For this review, take the finished solid that the model builds, in its own axes (mm). Round coordinates to 2 decimals unless told otherwise and drop trailing zeros. Order: outer loops, then holes, each group sorted by start corner. A loop starts at its lowest first (then second) coordinate and runs counter-clockwise, first axis right, second up. Notation, with made-up numbers: (-7.75, 53) - (29.25, 53) arc R14 cw to (29.25, 76) - close; hole circle Ø10 at (68, 24.5). An arc over 180 degrees is marked (long way). Write each question's results on one line, items separated by ' | '. Start each with the question number.
(1) Take a section at C-C, the plane x = 7.5. Give the boundary of the cut face in (y, z), plus the area to 3 significant figures.
(2) For L1, parallel to Z at x = -20.32, y = 0.15; L2, parallel to X at y = 0.4, z = 17.78; L3, parallel to X at y = -0.55, z = 15 (3 decimals), list the stretches that pass through material, from the lowest coordinate up. Write a range as from..to.
(3) Insertion check: pin 1 Ø4 at (x, z) = (-20.32, -17.78) entering from -Y; pin 2 Ø0.5 at (x, y) = (8, 0.5) entering from +Z; pin 3 Ø0.8 at (x, y) = (0, 0.5) entering from -Z; pin 4 Ø0.8 at (x, y) = (-7.5, 0) entering from -Z. Each pin has a flat end and moves straight along its axis. Give the tip position at first contact, or say it passes through.
(4) Take a section at B-B, the plane y = -0.4. Give the boundary of the cut face in (x, z) (3 decimals), plus the area to 3 significant figures.
(5) Take a section at A-A, the plane z = -14.5. Give the boundary of the cut face in (x, y) (3 decimals), plus the area to 3 significant figures.
```python
from build123d import *

# Parameters (mm, degrees)
SKETCH1_W             = 45.72
SKETCH1_H             = 40.64
BOSS_EXTRUDE1_DEPTH   = 0.762
FILLET1_R             = 2.54
F_4_CLEARANCE_HOLE1_D = 2.9464
SKETCH4_W             = 1.515
SKETCH4_H             = 4
CUT_EXTRUDE1_DEPTH    = 2.524


with BuildPart() as part:
    # Sketch1 → Boss-Extrude1 (new body, symmetric)
    with BuildSketch(Plane(origin=(0, 0, 0), x_dir=(1, 0, 0), z_dir=(0, 1, 0))):
        Rectangle(SKETCH1_W, SKETCH1_H)
    extrude(amount=BOSS_EXTRUDE1_DEPTH, both=True)

    # Fillet1
    fillet1_edges = [part.edges().sort_by_distance(p)[0] for p in [
        (22.86, 0, 20.32),
        (-22.86, 0, 20.32),
        (-22.86, 0, -20.32),
        (22.86, 0, -20.32),
    ]]
    fillet(fillet1_edges, radius=FILLET1_R)

    # #4 Clearance Hole1 (through all)
    with Locations(Plane(origin=(0, 0.762, 0), x_dir=(1, 0, 0), z_dir=(0, 1, 0))):
        with Locations((20.32, 17.78), (-20.32, -17.78), (-20.32, 17.78), (20.32, -17.78)):
            Hole(F_4_CLEARANCE_HOLE1_D / 2)

    # Sketch4 → Cut-Extrude1 (cut, through all)
    with BuildSketch(Plane(origin=(0, 0.762, 0), x_dir=(1, 0, 0), z_dir=(0, 1, 0))):
        Polygon((6.985, 16.32), (6.985, 20.32), (-6.985, 20.32), (-6.985, 16.32), (-6.985, 11.938), (6.985, 11.938), align=None)
        with Locations((7.7425, 18.32)):
            Rectangle(SKETCH4_W, SKETCH4_H)
        with Locations((-7.7425, 18.32)):
            Rectangle(SKETCH4_W, SKETCH4_H)
    cut_extrude1 = extrude(amount=-CUT_EXTRUDE1_DEPTH, mode=Mode.SUBTRACT)

    # Mirror1: Cut-Extrude1 across plane
    add(cut_extrude1.mirror(Plane.XY), mode=Mode.SUBTRACT)


solid = part.part
```
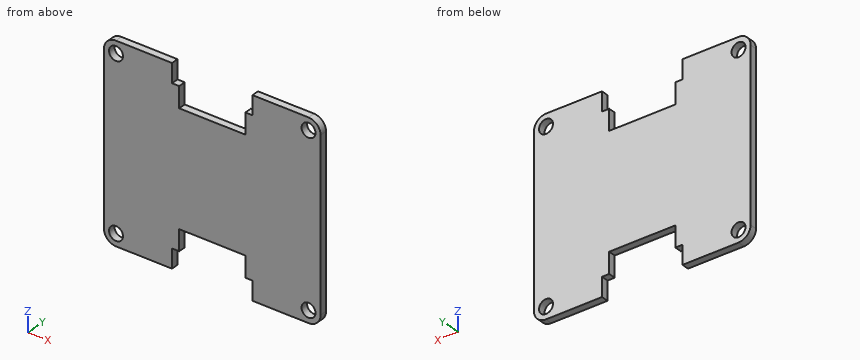
Results below:
1) outline: (-0.76, -16.32) - (0.76, -16.32) - (0.76, 16.32) - (-0.76, 16.32) - close | area: 49.7 mm^2
2) L1: z = -20.32..-19.25, -16.31..16.31, 19.25..20.32 | L2: x = -22.86..-21.79, -18.85..-8.5, 8.5..18.85, 21.79..22.86 | L3: x = -22.86..-6.985, 6.985..22.86
3) pin 1: stops at y = -0.76 | pin 2: stops at z = 16.32 | pin 3: stops at z = -11.94 | pin 4: stops at z = -16.32
4) outline: (-22.86, -17.78) arc R2.54 ccw to (-20.32, -20.32) - (-8.5, -20.32) - (-8.5, -16.32) - (-6.985, -16.32) - (-6.985, -11.938) - (6.985, -11.938) - (6.985, -16.32) - (8.5, -16.32) - (8.5, -20.32) - (20.32, -20.32) arc R2.54 ccw to (22.86, -17.78) - (22.86, 17.78) arc R2.54 ccw to (20.32, 20.32) - (8.5, 20.32) - (8.5, 16.32) - (6.985, 16.32) - (6.985, 11.938) - (-6.985, 11.938) - (-6.985, 16.32) - (-8.5, 16.32) - (-8.5, 20.32) - (-20.32, 20.32) arc R2.54 ccw to (-22.86, 17.78) - close; hole circle Ø2.946 at (-20.32, -17.78); hole circle Ø2.946 at (-20.32, 17.78); hole circle Ø2.946 at (20.32, -17.78); hole circle Ø2.946 at (20.32, 17.78) | area: 1,570 mm^2
5) outline: (-22.86, -0.762) - (-6.985, -0.762) - (-6.985, 0.762) - (-22.86, 0.762) - close; (6.985, -0.762) - (22.86, -0.762) - (22.86, 0.762) - (6.985, 0.762) - close | area: 48.4 mm^2
